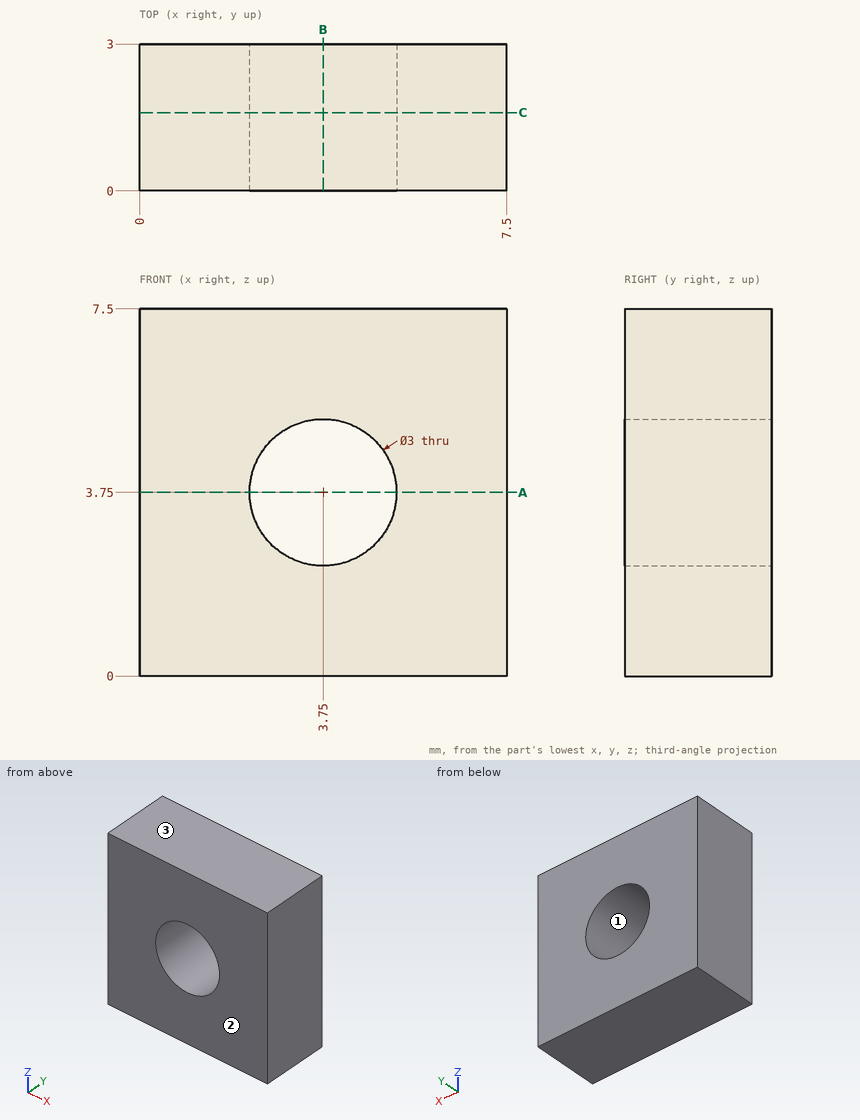
Could you check a few things on this drawing? It's one solid part, dimensions in mm from its lowest x, y, z. Coordinates: 2 decimals unless noted, no trailing zeros. Loops run counter-clockwise (first coordinate to the right, second up) from the corner with the lowest first, then second, coordinate; pieces in that order, holes last. Notation, with made-up numbers: (49.5, 59.25) - (98.5, 59.25) arc R26 ccw to (98.5, 88.25) - close; hole circle Ø6 at (-19.5, 57). An arc over 180 degrees is marked (long way). Answer as a JSON object with one key per item and string values. Group by question number.
Item 1: If we section it at A-A (z = 3.75): List the corners of the cut face in (x, y) for me, plus the area to 3 significant figures.
Item 2: If we section it at C-C (y = 1.6): List the corners of the cut face in (x, z) for me.
Item 3: If I drill on L1, parallel to Z at x = 3.75, y = 1.75; L2, parallel to Z at x = 3, y = 2.5, over which ranges is the centre line in solid material (lowest first)? Write a range as from..to.
Item 4: If we section it at B-B (x = 3.75): List the corners of the cut face in (y, z) for me, plus the area to 3 significant figures.
Item 5: If we mould it in two halves opening along Z, with no side actions, what happens to the marked faces 1, 2 and 3? For each: released by +Z, released by -Z, zero draft, split by the parting line, or undercut.
Returned:
{
 "1": {"outline": "(0, 0) - (2.25, 0) - (2.25, 3) - (0, 3) - close; (5.25, 0) - (7.5, 0) - (7.5, 3) - (5.25, 3) - close", "area": "13.5 mm²"},
 "2": {"outline": "(0, 0) - (7.5, 0) - (7.5, 7.5) - (0, 7.5) - close; hole circle Ø3 at (3.75, 3.75)"},
 "3": {"L1": "z = 0..2.25, 5.25..7.5", "L2": "z = 0..2.45, 5.05..7.5"},
 "4": {"outline": "(0, 0) - (3, 0) - (3, 2.25) - (0, 2.25) - close; (0, 5.25) - (3, 5.25) - (3, 7.5) - (0, 7.5) - close", "area": "13.5 mm²"},
 "5": {"face 1": "undercut", "face 2": "zero draft", "face 3": "released by +Z"}
}
